Part model, mm, in its own coordinate system. Face numbers are marked on the shaded views. A direction names the side the tool comes from. Round coordinates to 2 decimals unless told otherwise and drop trailing zeros. Loops run counter-clockwise (first coordinate to the right, second up) from the corner with the lowest first, then second, coordinate; pieces in that order, holes last.
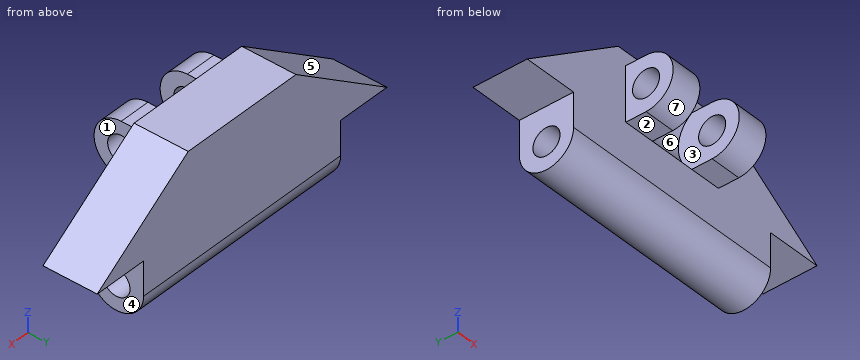
from build123d import *

# Parameters (mm, degrees)
BOSS_EXTRUDE1_DEPTH      = 4
BOSS_EXTRUDE2_START      = 4
SKETCH2_R                = 1
BOSS_EXTRUDE2_DEPTH      = 17
BOSS_EXTRUDE3_DEPTH      = 4
BOSS_EXTRUDE3_DEPTH_BACK = 4
BOSS_EXTRUDE3_START      = 12.5
SKETCH3_R                = 1
CUT_EXTRUDE1_REACH       = 29.221
SKETCH4_W                = 3.4
SKETCH4_H                = 3.5
CUT_EXTRUDE2_DEPTH       = 3.4


with BuildPart() as part:
    # Sketch1 → Boss-Extrude1 (new body)
    with BuildSketch(Plane(origin=(0, 0, 0), x_dir=(1, 0, 0), z_dir=(0, 1, 0))):
        Polygon((0, 0), (7.854814037, -5.5), (17.145185963, -5.5), (25, 0), align=None)
    extrude(amount=BOSS_EXTRUDE1_DEPTH)

    # Sketch2 → Boss-Extrude2 (add)
    with BuildSketch(Plane(origin=(0, 0, 0), x_dir=(0, 0, -1), z_dir=(1, 0, 0)).offset(BOSS_EXTRUDE2_START)):
        with BuildLine():
            Line((0, 0), (2.5, 0))
            ThreePointArc((2.5, 0), (4.5, 2), (2.5, 4))
            Line((2.5, 4), (0, 4))
            Line((0, 4), (0, 0))
        make_face()
        with Locations((2.5, 2)):
            Circle(SKETCH2_R, mode=Mode.SUBTRACT)
    extrude(amount=BOSS_EXTRUDE2_DEPTH)

    # Sketch3 → Boss-Extrude3 (add, two sides: drawn at the far end of the back side and taken through both)
    with BuildSketch(Plane(origin=(0, 0, 0), x_dir=(0, 0, -1), z_dir=(1, 0, 0)).offset(BOSS_EXTRUDE3_START - BOSS_EXTRUDE3_DEPTH_BACK)):
        with BuildLine():
            Line((-4.5, 0), (-0.5, 0))
            Line((-0.5, 0), (-0.5, -1.5))
            ThreePointArc((-0.5, -1.5), (-2.5, -3.5), (-4.5, -1.5))
            Line((-4.5, -1.5), (-4.5, 0))
        make_face()
        with Locations((-2.5, -1.5)):
            Circle(SKETCH3_R, mode=Mode.SUBTRACT)
    extrude(amount=BOSS_EXTRUDE3_DEPTH + BOSS_EXTRUDE3_DEPTH_BACK)

    # Sketch4 → Cut-Extrude1 (cut, up to next)
    with BuildSketch(Plane.XY.offset(5.5), mode=Mode.PRIVATE) as cut_extrude1_sk1:
        with Locations((12.5, -1.75)):
            Rectangle(SKETCH4_W, SKETCH4_H)
    cut_extrude1_tool1 = extrude(cut_extrude1_sk1.sketch, amount=-CUT_EXTRUDE1_REACH, mode=Mode.PRIVATE) & part.part
    add(cut_extrude1_tool1.solids().sort_by_distance((12.5, -1.75, 5.5))[0], mode=Mode.SUBTRACT)

    # Sketch5 → Cut-Extrude2 (cut)
    with BuildSketch(Plane.ZY.offset(-14.2)):
        with BuildLine():
            Line((4.5, 0), (0.5, 0))
            ThreePointArc((0.5, 0), (2.5, 1), (4.5, 0))
        make_face()
    extrude(amount=CUT_EXTRUDE2_DEPTH, mode=Mode.SUBTRACT)


solid = part.part
1) Slice it at B-B, the plane z = 3. Give the cut face in (x, y), then the cut area to 3 significant figures.
Values:
outline: (4.28, 0) - (8.5, 0) - (8.5, -0.63) - (10.8, -0.63) - (10.8, 0.95) - (14.2, 0.95) - (14.2, -0.63) - (16.5, -0.63) - (16.5, 0) - (20.72, 0) - (20.72, 4) - (4.28, 4) - close; (8.5, -3.44) - (10.8, -3.44) - (10.8, -2.37) - (8.5, -2.37) - close; (14.2, -3.44) - (16.5, -3.44) - (16.5, -2.37) - (14.2, -2.37) - close
area: 70.3 mm2
2) Slice it at A-A, the plane y = 2. Give the cut face in (x, z).
Values:
outline: (0, 0) - (4, 0) - (4, -1.5) - (21, -1.5) - (21, 0) - (25, 0) - (17.15, 5.5) - (7.85, 5.5) - close; (4, -4.5) - (21, -4.5) - (21, -3.5) - (4, -3.5) - close
3) Wall check: line 1 along Y through (x, z) = (16, -2.5); line 2 along Y through (x, z) = (15.55, 2.5); line 3 along Z through (x, y) = (15.95, -1.5). Give the ranges that are in metal, low to high.
Values:
line 1: y = 0 to 1, 3 to 4
line 2: y = -3.5 to -2.5, -0.5 to 4
line 3: z = 0.5 to 1.5, 3.5 to 4.5
4) Drop flat-ended pins along their axis: pin 1 Ø3 at (y, z) = (2.5, -3) entering from -X; pin 2 Ø4 at (y, z) = (-2.5, 2) entering from -X; pin 3 Ø3 at (y, z) = (-1, 3) entering from +X. Give the stop position or say it passes through.
Values:
pin 1: stops at x = 4
pin 2: stops at x = 8.5
pin 3: stops at x = 22.31
5) Tool access for the marked faces 1, 2, 3 and 4: list every direction of +Z, -Z, +X, -X, +Y, -Y with a clear straight run to the whole face (end or side of a thin tool).
Values:
face 1: +Z, -Z, +X, -Y
face 2: -Z, +X, -X, -Y
face 3: -Y
face 4: -Z, +X, +Y, -Y
6) Mould opens along Z. For the marked faces 5, 6 and 7 say: released by +Z, released by -Z, zero draft, split by the parting line, or undercut.
Values:
face 5: released by +Z
face 6: undercut
face 7: split by the parting line
7) Slice it at C-C, the plane y = -1.25. Give the cut face in (x, z), then the cut area to 3 significant figures.
Values:
outline: (8.5, 0.5) - (10.8, 0.5) - (10.8, 1.53) - (8.5, 1.53) - close; (8.5, 3.47) - (10.8, 3.47) - (10.8, 4.5) - (8.5, 4.5) - close; (14.2, 0.5) - (16.5, 0.5) - (16.5, 1.53) - (14.2, 1.53) - close; (14.2, 3.47) - (16.5, 3.47) - (16.5, 4.5) - (14.2, 4.5) - close
area: 9.49 mm2
8) Slice it at D-D, the plane x = 6.75. Give the cut face in (y, z), then the cut area to 3 significant figures.
Values:
outline: (0, -2.5) arc R2 ccw to (4, -2.5) - (4, 4.73) - (0, 4.73) - close; hole circle Ø2 at (2, -2.5)
area: 32.0 mm2
